```python
from build123d import *

# Parameters (mm, degrees)
ESQUISSE1_R      = 5.5
EXTRUSION1_DEPTH = 12
CHANFREIN1_SIZE  = 0.5
CHANFREIN2_SIZE  = 0.5


with BuildPart() as part:
    # Esquisse1 → Extrusion1 (new, symmetric)
    with BuildSketch(Plane.XY):
        Circle(ESQUISSE1_R)
    extrude(amount=EXTRUSION1_DEPTH, both=True)

    # Chanfrein1
    chanfrein1_edges = [part.edges().sort_by_distance(p)[0] for p in [
        (-5.5, 0, 12),
    ]]
    chamfer(chanfrein1_edges, length=CHANFREIN1_SIZE)

    # Chanfrein2
    chanfrein2_edges = [part.edges().sort_by_distance(p)[0] for p in [
        (-5.5, 0, -12),
    ]]
    chamfer(chanfrein2_edges, length=CHANFREIN2_SIZE)

    # Esquisse3 → Gorge pour ANSI B27.8M - 3DM1-11, Circlip haut rendement1 (revolve, cut)
    with BuildSketch(Plane(origin=(0, 0, 24), x_dir=(0, 1, 0), z_dir=(-1, 0, 0)), mode=Mode.PRIVATE) as gorge_pour_ansi_b27_8m_3dm1_11_circli_sk:
        with BuildLine():
            Line((5.25, 13), (6.6, 13))
            Line((6.6, 13), (6.6, 14))
            Line((6.6, 14), (5.25, 14))
            ThreePointArc((5.25, 14), (5.179289322, 13.970710678), (5.15, 13.9))
            Line((5.15, 13.9), (5.15, 13.1))
            ThreePointArc((5.15, 13.1), (5.179289322, 13.029289322), (5.25, 13))
        make_face()
    gorge_pour_ansi_b27_8m_3dm1_11_circli = revolve(gorge_pour_ansi_b27_8m_3dm1_11_circli_sk.sketch.rotate(Axis((0, 0, 74), (0, 0, -1)), 270), axis=Axis((0, 0, 74), (0, 0, -1)), mode=Mode.SUBTRACT)

    # Symétrie1: Gorge pour ANSI B27.8M - 3DM1-11, Circlip haut rendement1 across plane
    add(gorge_pour_ansi_b27_8m_3dm1_11_circli.mirror(Plane.XY), mode=Mode.SUBTRACT)


solid = part.part
```
Work out the finished part from the listing and answer in its coordinate system (mm). A direction names the side the tool comes from. Give positions to 0.01 mm unless a question says otherwise; leave off trailing zeros. Write each loop counter-clockwise with the first axis right and the second up, starting at its lowest first coordinate (ties: lowest second). Pieces come first, ordered by that corner, then holes.
(1) Flat-ended cylindrical pins translate along their axes: pin 1 Ø2 at (y, z) = (-2.5, -3) entering from +X; pin 2 Ø6 at (y, z) = (0.5, 8.5) entering from +X. Find the tip coordinate at first contact, or state that the pin passes through.
Final values:
pin 1: stops at x = 5.29
pin 2: stops at x = 5.5
(2) Which of the six approach directions +Z, -Z, +X, -X, +Y, -Y give full straight-line access (tool end or side, diameter ignored) to faces 4 (the flat face through (0, 0, -12)), 5 (the cylindrical face through (1.116, -5.028, 10.506))?
Final values:
face 4: -Z, +X, -X, +Y, -Y
face 5: none
(3) Straight lines are drawn through the part: line 1 (Y direction, x = -0.25, z = -1.25); line 2 (Y direction, x = 2.25, z = 7); line 3 (X direction, y = -2.75, z = 4.75). For each, find the intervals that lie inside material, in ascending order.
Final values:
line 1: y = -5.49 to 5.49
line 2: y = -5.02 to 5.02
line 3: x = -4.76 to 4.76
(4) The mould has two halves that part along Z. Classify faces 1 (the cylindrical face through (-1.19, -5.37, -11.25)), 2 (the flat face through (0, 0, 12)), 3 (the cylindrical face through (1.116, -5.028, -10.506)): pulls with the +Z half, pulls with the -Z half, needs draft (parallel to the pull), parting line crosses it, or undercut.
Final values:
face 1: needs draft
face 2: pulls with the +Z half
face 3: undercut
(5) The part is cut by section A-A on z = -6. Write down the section's boundary in (x, y), plus the area to 3 significant figures.
Final values:
outline: circle Ø11 at (0, 0)
area: 95.0 mm2
